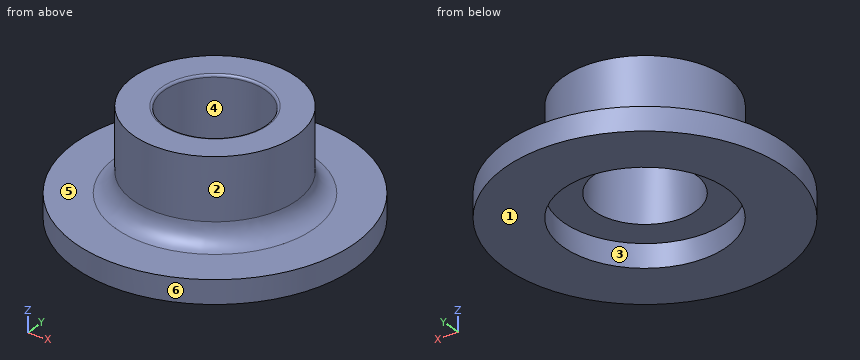
```python
from build123d import *

# Parameters (mm, degrees)
F0_R     = 12
F0_R_2   = 7
F1_DEPTH = 2
F0_R_3   = 4.35
F2_DEPTH = 7.021
F8_R     = 0.2


with BuildPart() as f1:
    # F0 (on Top) → F1 (new body)
    with BuildSketch(Plane.XY):
        Circle(F0_R)
        Circle(F0_R_2, mode=Mode.SUBTRACT)
    extrude(amount=-F1_DEPTH)

    # F0 (on Top) → F2 (join)
    with BuildSketch(Plane.XY):
        Circle(F0_R_2)
        Circle(F0_R_3, mode=Mode.SUBTRACT)
    extrude(amount=F2_DEPTH)

    # F6 (on Front) → F7 (revolve)
    with BuildSketch(Plane.XZ):
        with BuildLine():
            ThreePointArc((-7, 1.7562480825), (-7.4708650568, 0.639716712), (-8.5, 0))
            Line((-8.5, 0), (-7, 0))
            Line((-7, 0), (-7, 1.7562480825))
        make_face()
    revolve(axis=Axis((0, 0, 5.6352536849), (0, 0, 1)))

    # F8
    f8_edges = [f1.edges().sort_by_distance(p)[0] for p in [
        (-4.35, 0, 7.021),
    ]]
    fillet(f8_edges, radius=F8_R)


solid = f1.part
```
The model under review builds one solid part; all positions refer to its coordinate system, in mm. Face numbers are marked on the shaded views. A direction names the side the tool comes from. Coordinates: 2 decimals unless noted, no trailing zeros. Write each loop counter-clockwise with the first axis right and the second up, starting at its lowest first coordinate (ties: lowest second). Pieces come first, ordered by that corner, then holes.
1) Clearance check with flat-ended pins moving along their axes: pin 1 Ø4 at (x, y) = (3, 1) entering from -Z; pin 2 Ø2 at (y, z) = (-3.5, 0.5) entering from +X; pin 3 Ø5 at (y, z) = (-2, 3.5) entering from -X. State where each tip first meets the part, or that it passes through.
2) Machinability: for the marked faces 1, 2 and 3, which of the approach directions +Z, -Z, +X, -X, +Y, -Y give a long, thin tool a straight path to every point of the face, cutting with its end or side? Answer none if there is none.
3) We need section C-C on z = 6.25. State the section outline as (x, y) points, then the cut area to 3 significant figures.
4) We need section A-A on y = 0. State the section outline as (x, z) points, then the cut area to 3 significant figures.
5) The part is to be moulded in two halves that separate along Y. For the marked faces 4, 5 and 6, say which applies: pulls with the +Y half, pulls with the -Y half, needs draft (parallel to the pull), parting line crosses it, or undercut.
6) To check wall thickness, follow probe 1 along Y at (x, z) = (0, -1.2); probe 2 along Y at (x, z) = (0, 2.75); probe 3 along Z at (x, y) = (9.75, 6.5). State the ranges of each line that lie inside material, in increasing order.
Answer list:
1. pin 1: stops at z = 0
1. pin 2: stops at x = 11.71
1. pin 3: stops at x = -7.06
2. face 1: -Z, +X, -X, +Y, -Y
2. face 2: +Z
2. face 3: -Z
3. outline: circle Ø14 at (0, 0); hole circle Ø8.7 at (0, 0)
3. area: 94.5 mm2
4. outline: (-12, -2) - (-7, -2) - (-7, 0) - (-4.35, 0) - (-4.35, 6.82) arc R0.2 ccw to (-4.55, 7.02) - (-7, 7.02) - (-7, 1.76) arc R2 cw to (-8.5, 0) - (-12, 0) - close; (4.35, 0) - (7, 0) - (7, -2) - (12, -2) - (12, 0) - (8.5, 0) arc R2 cw to (7, 1.76) - (7, 7.02) - (4.55, 7.02) arc R0.2 ccw to (4.35, 6.82) - close
4. area: 58.7 mm2
5. face 4: undercut
5. face 5: needs draft
5. face 6: parting line crosses it
6. probe 1: y = -12 to -7, 7 to 12
6. probe 2: y = -7 to -4.35, 4.35 to 7
6. probe 3: z = -2 to 0
